Check sheet for the modelled part. Datum: model origin and axes. Units: mm. A direction names the side the tool comes from. Round coordinates to 2 decimals unless told otherwise and drop trailing zeros. Order: outer loops, then holes, each group sorted by start corner. A loop starts at its lowest first (then second) coordinate and runs counter-clockwise, first axis right, second up.
```python
from build123d import *

# Parameters (mm, degrees)
F1_DEPTH = 16
F2_R     = 1.99999
F3_SIZE  = 0.8
F4_SIZE  = 0.6


# Not quite as in the source:
# - a fillet or chamfer is up to 0.001 mm smaller than in the source, because OpenCascade refuses the exact size


with BuildPart() as f1:
    # F0 (on Front) → F1 (new body)
    with BuildSketch(Plane.XZ):
        with BuildLine():
            ThreePointArc((7.8, 0), (7.3700465154, -2.5539017916), (6.1275860612, -4.82625))
            Line((6.1275860612, -4.82625), (0.648940015, -11.7821422864))
            ThreePointArc((0.648940015, -11.7821422864), (5.4420247731, -10.4701655368), (9.2699378875, -7.30125))
            ThreePointArc((9.2699378875, -7.30125), (11.1495575489, -3.8635950181), (11.8, 0))
            ThreePointArc((11.8, 0), (-4.0644802866, 11.0779059393), (-9, -7.6315136113))
            Line((-9, -7.6315136113), (-5.9491525424, -5.0445598448))
            ThreePointArc((-5.9491525424, -5.0445598448), (-2.6866903589, 7.322683587), (7.8, 0))
        make_face()
        with BuildLine():
            ThreePointArc((9.2699378875, -7.30125), (5.4420247731, -10.4701655368), (0.648940015, -11.7821422864))
            Line((0.648940015, -11.7821422864), (-9.4270554788, -24.575))
            ThreePointArc((-9.4270554788, -24.575), (-5.5744413376, -21.3733540676), (-0.7504354082, -20.0234877073))
            Line((-0.7504354082, -20.0234877073), (9.2699378875, -7.30125))
        make_face()
        with BuildLine():
            ThreePointArc((-0.7504354082, -20.0234877073), (-5.5744413376, -21.3733540676), (-9.4270554788, -24.575))
            ThreePointArc((-9.4270554788, -24.575), (-3.9290796794, -43.3385331006), (12, -32))
            ThreePointArc((12, -32), (11.4891252931, -28.5358983849), (10, -25.3667504193))
            Line((10, -25.3667504193), (6.6666666667, -27.5778336129))
            ThreePointArc((6.6666666667, -27.5778336129), (7.6594168621, -29.6905989232), (8, -32))
            ThreePointArc((8, -32), (-2.619386453, -39.559022067), (-6.2847036525, -27.05))
            Line((-6.2847036525, -27.05), (-0.7504354082, -20.0234877073))
        make_face()
        with BuildLine():
            Line((0.648940015, -11.7821422864), (6.1275860612, -4.82625))
            ThreePointArc((6.1275860612, -4.82625), (0.1409766904, -7.7987258942), (-5.9491525424, -5.0445598448))
            Line((-5.9491525424, -5.0445598448), (-9, -7.6315136113))
            ThreePointArc((-9, -7.6315136113), (-4.6628296471, -10.8396503487), (0.648940015, -11.7821422864))
        make_face()
    extrude(amount=F1_DEPTH)

    # F2 (radius 2 in the source; OpenCascade refuses exactly that, so slightly less here)
    f2_edges = [f1.edges().sort_by_distance(p)[0] for p in [
        (6.127586, -8, -4.82625),
        (9.269938, -8, -7.30125),
        (10, -8, -25.36675),
        (6.666667, -8, -27.577834),
        (0.64894, -8, -11.782142),
    ]]
    fillet(f2_edges, radius=F2_R)

    # F3
    f3_edges = [f1.edges().sort_by_distance(p)[0] for p in [
        (-6.127586, -16, 4.82625),
        (-6.127586, 0, 4.82625),
    ]]
    chamfer(f3_edges, length=F3_SIZE)

    # F4
    f4_edges = [f1.edges().sort_by_distance(p)[0] for p in [
        (-3.880931, -16, 11.143535),
        (1.492617, 0, -17.175625),
        (-5.523718, 0, -19.619177),
        (-1.302823, 0, -12.768079),
        (-1.69128, 0, -43.880218),
        (-3.880931, 0, 11.143535),
        (9.862297, 0, -26.340194),
        (8.164968, 0, -26.583973),
        (-1.127522, 0, -39.920145),
        (7.360063, 0, -27.658852),
        (-5.523718, -16, -19.619177),
        (-1.302823, -16, -12.768079),
        (-1.69128, -16, -43.880218),
        (9.862297, -16, -26.340194),
        (1.492617, -16, -17.175625),
        (8.164968, -16, -26.583973),
        (-1.127522, -16, -39.920145),
        (7.360063, -16, -27.658852),
    ]]
    chamfer(f4_edges, length=F4_SIZE)


solid = f1.part
```
Item 1: Release check for a two-part mould opening along X. For faces 5 (the flat face through (1, 0, -16)), 6 (the cylindrical face through (9.89, -8.1, -26.35)), 7 (the flat face through (-5.23, -15.704, -19.738)) record: released by +X, released by -X, zero draft, split by the parting line, or undercut.
Answer:
face 5: zero draft
face 6: undercut
face 7: released by -X
Item 2: Sectioned sample at B-B (x = 0). Record the cut outline in (y, z).
Answer:
outline: (-16, -43.4) - (-15.4, -44) - (-0.6, -44) - (0, -43.4) - (0, -40.6) - (-0.6, -40) - (-15.4, -40) - (-16, -40.6) - close; (-16, -18.1) - (-15.4, -19.07) - (-0.6, -19.07) - (0, -18.1) - (0, -8.6) - (-0.8, -7.8) - (-15.2, -7.8) - (-16, -8.6) - close; (-16, 8.6) - (-15.2, 7.8) - (-0.8, 7.8) - (0, 8.6) - (0, 11.2) - (-0.6, 11.8) - (-15.4, 11.8) - (-16, 11.2) - close
Item 3: Sectioned sample at C-C (z = -18). Record the cut outline in (x, y).
Answer:
outline: (-4.25, -15.4) - (-3.48, -16) - (0.08, -16) - (0.84, -15.4) - (0.84, -0.6) - (0.08, 0) - (-3.48, 0) - (-4.25, -0.6) - close
Item 4: Go/stop test with flat-tipped pins: P1, Ø5, axis at x = -8, y = -4.5, coming from the -Z side; P2, Ø4, axis at y = -14, z = -6, coming from the -X side. Record where each tip stops, or that it passes through.
Answer:
P1: stops at z = -42.67
P2: stops at x = -11.1
Item 5: Scan lines: line 1 along X through (y, z) = (-7.5, -32); line 2 along Z through (x, y) = (0, -9.75); line 3 along Z through (x, y) = (2, -1.75). Record each from-to range of solid material in increasing order.
Answer:
line 1: x = -12 to -8, 8 to 12
line 2: z = -44 to -40, -19.07 to -7.8, 7.8 to 11.8
line 3: z = -43.83 to -39.75, -16.53 to -7.54, 7.54 to 11.63
Item 6: Access from +Z, -Z, +X, -X, +Y, -Y to the whole of each face (thin tool, end or side, straight path). Record for faces 1 (the flat face through (1, -16, -16)), 2 (the flat face through (-5.47, -7.9, -19.55)), 3 (the cylindrical face through (7.366, -8.104, -27.641)), 4 (the flat face through (-5.237, -0.304, -19.733)).
Answer:
face 1: +Z, -Z, +X, -X, -Y
face 2: -X, +Y, -Y
face 3: +Y, -Y
face 4: -X, +Y
